```python
from build123d import *

# Parameters (mm, degrees)
SKETCH3_R          = 40
CUT_EXTRUDE1_DEPTH = 10


with BuildPart() as part:
    # Sketch1 → Loft1 section 0
    with BuildSketch(Plane(origin=(0, 0, 0), x_dir=(0, 0, -1), z_dir=(1, 0, 0))):
        with BuildLine():
            Line((0, 0), (-350, 0))
            Line((-350, 0), (-350, 75))
            Line((-350, 75), (-250, 200))
            Line((-250, 200), (0, 200))
            Line((0, 200), (0, 0))
        make_face()
    # Sketch2 → Loft1 section 1
    with BuildSketch(Plane(origin=(100, 0, 0), x_dir=(0, 0, -1), z_dir=(1, 0, 0))):
        with BuildLine():
            Line((0, 0), (4.422435972, 200))
            Line((4.422435972, 200), (-195.577564028, 200))
            Line((-195.577564028, 200), (-300, 75))
            Line((-300, 75), (-300, 0))
            Line((-300, 0), (0, 0))
        make_face()
    loft1 = loft()

    # Sketch3 → Cut-Extrude1 (cut)
    with BuildSketch(Plane(origin=(100, 0, 0), x_dir=(0, 0, -1), z_dir=(1, 0, 0))):
        with Locations((-220, 0)):
            Circle(SKETCH3_R)
        with Locations((-70, 0)):
            Circle(SKETCH3_R)
    cut_extrude1 = extrude(amount=-CUT_EXTRUDE1_DEPTH, mode=Mode.SUBTRACT)

    # Mirror2: Loft1, Cut-Extrude1 across plane
    add(loft1.mirror(Plane.ZY))
    add(cut_extrude1.mirror(Plane.ZY), mode=Mode.SUBTRACT)


solid = part.part
```
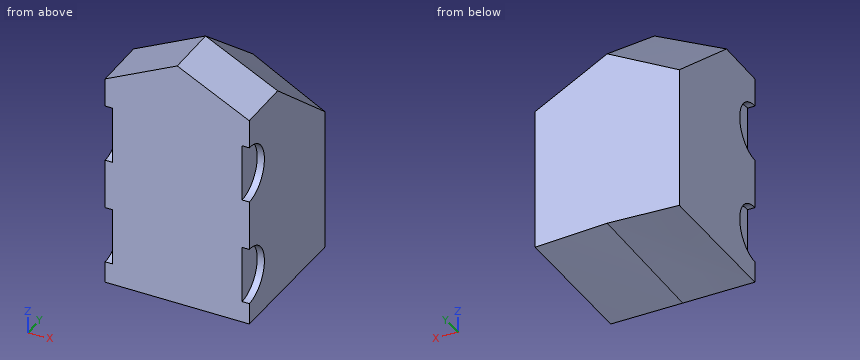
The listing builds one solid part. Answer for the finished solid, in the listing's coordinates (mm). Round coordinates to 2 decimals unless told otherwise and drop trailing zeros. Order: outer loops, then holes, each group sorted by start corner. A loop starts at its lowest first (then second) coordinate and runs counter-clockwise, first axis right, second up. Notation, with made-up numbers: (86.25, 30) -> (115.25, 30) arc R37 cw to (115.25, 66) -> close; hole circle Ø9 at (11, 9). An arc over 180 degrees is marked (long way). Answer as CSV lines item,"result". Start each with the question number.
(1) Flat-ended cylindrical pins translate along their axes: pin 1 Ø4 at (x, y) = (-5.5, 108.5) entering from +Z; pin 2 Ø1.5 at (y, z) = (32.5, 203) entering from +X; pin 3 Ø2 at (x, z) = (-71, 300.5) entering from +Y. Find the tip coordinate at first contact, or state that the pin passes through.
(2) Find the intervals of material crossed by probe 1 along X at (y, z) = (31, 47); probe 2 along Z at (x, y) = (-19, 57); probe 3 along Y at (x, z) = (-39, 299), in increasing order. Write a range as from..to.
(3) The part is cut by section A-A (z = 70). Determine the outline of the cut face in (x, y).
Evaluation:
1,pin 1,"z = 322.29"
1,pin 2,"x = 90"
1,pin 3,"y = 93.33"
2,probe 1,"-90..90"
2,probe 2,"-0.24..340.5"
2,probe 3,"0..113.71"
3,outline,"(-100, 40) -> (-90, 40) -> (-90, 0) -> (90, 0) -> (90, 40) -> (100, 40) -> (100, 200) -> (-100, 200) -> close"
